Could you check a few things on this drawing? It's one solid part, dimensions in mm from its lowest x, y, z. A direction names the side the tool comes from. Round coordinates to 2 decimals unless told otherwise and drop trailing zeros. Write each loop counter-clockwise with the first axis right and the second up, starting at its lowest first coordinate (ties: lowest second). Pieces come first, ordered by that corner, then holes. Notation, with made-up numbers: (21.5, 79.5) -> (56.5, 79.5) arc R30 cw to (56.5, 112.5) -> close; hole circle Ø6 at (76.25, 75). An arc over 180 degrees is marked (long way). Put each result on its own line as item: value. Start each with the question number.
1) I want a section at A-A, the plane x = 22.5. List the corners of the cut face in (y, z) for me, then the cut area to 3 significant figures.
2) I want a section at B-B, the plane x = 40.5. List the corners of the cut face in (y, z) for me, then the cut area to 3 significant figures.
3) I want a section at C-C, the plane z = 27.5. List the corners of the cut face in (x, y) for me.
4) I want a section at D-D, the plane y = 2.75. List the corners of the cut face in (x, z) for me.
5) Which directions (+Z, -Z, +X, -X, +Y, -Y) give clear straight access to the entire face, cutting with the end or side of a thin tool? Please do the marked faces 3, 4 and 5.
6) If I drill on line 1 along X through (y, z) = (0.9, 27.5); line 2 along Z through (x, y) = (22.5, 1.25); line 3 along Z through (x, y) = (40.5, 0.45), over which ranges is the centre line in solid material (lowest first)? Write a range as [from, to].
7) We'd pull the mould along X, two halves only. Please class the marked faces 1 and 2: released by +X, released by -X, zero draft, split by the parting line, or undercut.
8) Will these pins go through, and if not, where does the flat tip stop? P1, Ø4.5, axis at x = 9, z = 26.5, coming from the +Y side; P2, Ø3, axis at y = 4.5, z = 33, coming from the -X side; P3, Ø2, axis at x = 37.5, y = 1.5, coming from the -Z side; P4, Ø1.8, axis at x = 4.5, z = 27.5, coming from the -Y side.
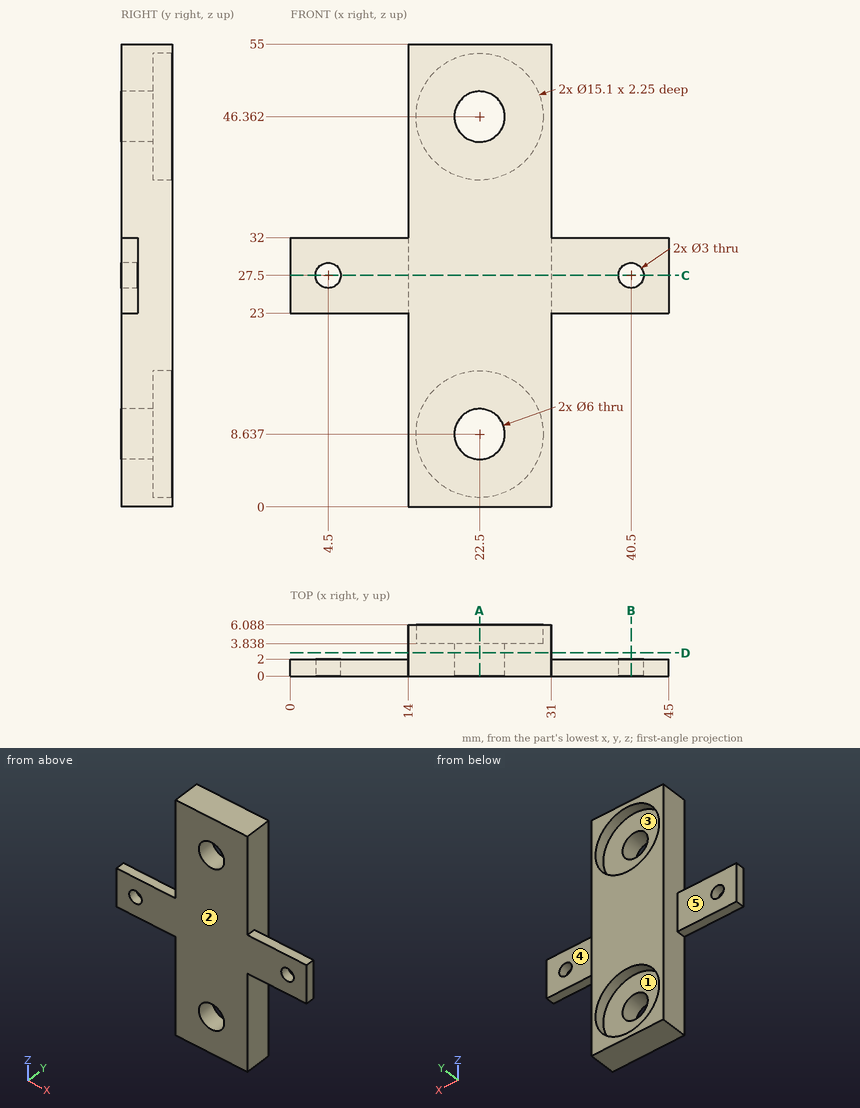
Findings:
1. outline: (0, 0) -> (6.09, 0) -> (6.09, 1.09) -> (3.84, 1.09) -> (3.84, 5.64) -> (0, 5.64) -> close; (0, 11.64) -> (3.84, 11.64) -> (3.84, 16.19) -> (6.09, 16.19) -> (6.09, 38.81) -> (3.84, 38.81) -> (3.84, 43.36) -> (0, 43.36) -> close; (0, 49.36) -> (3.84, 49.36) -> (3.84, 53.91) -> (6.09, 53.91) -> (6.09, 55) -> (0, 55) -> close
1. area: 221 mm2
2. outline: (0, 23) -> (2, 23) -> (2, 26) -> (0, 26) -> close; (0, 29) -> (2, 29) -> (2, 32) -> (0, 32) -> close
2. area: 12.0 mm2
3. outline: (0, 0) -> (3, 0) -> (3, 2) -> (0, 2) -> close; (6, 0) -> (39, 0) -> (39, 2) -> (31, 2) -> (31, 6.09) -> (14, 6.09) -> (14, 2) -> (6, 2) -> close; (42, 0) -> (45, 0) -> (45, 2) -> (42, 2) -> close
4. outline: (14, 0) -> (31, 0) -> (31, 55) -> (14, 55) -> close; hole circle Ø6 at (22.5, 8.64); hole circle Ø6 at (22.5, 46.36)
5. face 3: +Y
5. face 4: +Z, -Z, +X, +Y
5. face 5: +Z, -Z, -X, +Y
6. line 1: x = [0, 3], [6, 39], [42, 45]
6. line 2: z = [0, 5.64], [11.64, 43.36], [49.36, 55]
6. line 3: z = [23, 26], [29, 32]
7. face 1: undercut
7. face 2: zero draft
8. P1: stops at y = 2
8. P2: stops at x = 14
8. P3: stops at z = 23
8. P4: passes through
